Read the model definition and answer for the solid it produces. Units are mm, in the model's axes. A direction names the side the tool comes from. Coordinates: 2 decimals unless noted, no trailing zeros. Write each loop counter-clockwise with the first axis right and the second up, starting at its lowest first coordinate (ties: lowest second). Pieces come first, ordered by that corner, then holes.
Item 1: Straight lines are drawn through the part: probe 1 along Y at (x, z) = (0, 30); probe 2 along X at (y, z) = (-0.75, 15); probe 3 along Z at (x, y) = (-1.5, -0.75). For each, find the intervals that lie inside material, in ascending order.
Item 2: Determine the mould class of faces 4 (the face through (1.926, 0.607, 24.417)), 5 (the face through (0, 0, 12.827)), 6 (the face through (5.474, -3.219, 22.874)), 7 (the face through (0, 0, 0)) for opening direction Y: released by +Y, released by -Y, zero draft, split by the parting line, or undercut.
Item 3: Section C-C (y = -5.25) is taken. Give the vertices of the cut face in (x, z).
Item 4: Section D-D (x = -6) is taken. Give the vertices of the cut face in (y, z).
Item 5: Section A-A (z = 18.5) is taken. Give the vertices of the cut face in (x, y), then the cut area to 3 significant figures.
Item 6: A tool of negligible diameter and unlimited length cuts with its end or side. For faces 1 (the face through (5.525, 3.131, 22.874)), 2 (the face through (0, -6.35, 23)), 3 (the face through (-5.525, -3.131, 22.874)), from which of +Z, -Z, +X, -X, +Y, -Y can it reach the whole face along a straight path? Write none if from no direction.
Item 7: Each of these flat-tipped pins is pushed along its axis until it touches: P1, Ø3, axis at x = 0, y = 0, coming from the +Z side; P2, Ø3, axis at y = 5, z = 6, coming from the +X side; P3, Ø4, axis at x = 4.5, z = 22.5, coming from the +Y side. Where does it stop, or does it pass through?
Item 8: Section B-B (x = 0) is taken. Give the vertices of the cut face in (y, z).
from build123d import *

# Parameters (mm, degrees)
SKETCH2_R           = 7.9248
BOSS_EXTRUDE1_DEPTH = 10.414
BOSS_EXTRUDE2_DEPTH = 25.273
SKETCH4_R           = 2.0193
CUT_EXTRUDE1_DEPTH  = 22.86


with BuildPart() as part:
    # Sketch2 → Boss-Extrude1 (new body)
    with BuildSketch(Plane.XY):
        Circle(SKETCH2_R)
    extrude(amount=BOSS_EXTRUDE1_DEPTH)

    # Sketch3 → Boss-Extrude2 (add)
    with BuildSketch(Plane.XY.offset(10.414)):
        Polygon((7.332348419, 0), (3.666174209, 6.35), (-3.666174209, 6.35), (-7.332348419, 0), (-3.666174209, -6.35), (3.666174209, -6.35), align=None)
    extrude(amount=BOSS_EXTRUDE2_DEPTH)

    # Sketch4 → Cut-Extrude1 (cut)
    with BuildSketch(Plane.XY.offset(35.687)):
        Circle(SKETCH4_R)
    extrude(amount=-CUT_EXTRUDE1_DEPTH, mode=Mode.SUBTRACT)


solid = part.part
Established:
1. probe 1: y = -6.35 to -2.02, 2.02 to 6.35
1. probe 2: x = -6.9 to -1.87, 1.87 to 6.9
1. probe 3: z = 0 to 12.83
2. face 4: undercut
2. face 5: undercut
2. face 6: released by -Y
2. face 7: zero draft
3. outline: (-5.94, 0) - (5.94, 0) - (5.94, 10.41) - (4.3, 10.41) - (4.3, 35.69) - (-4.3, 35.69) - (-4.3, 10.41) - (-5.94, 10.41) - close
4. outline: (-5.18, 0) - (5.18, 0) - (5.18, 10.41) - (2.31, 10.41) - (2.31, 35.69) - (-2.31, 35.69) - (-2.31, 10.41) - (-5.18, 10.41) - close
5. outline: (-7.33, 0) - (-3.67, -6.35) - (3.67, -6.35) - (7.33, 0) - (3.67, 6.35) - (-3.67, 6.35) - close; hole circle Ø4.04 at (0, 0)
5. area: 127 mm2
6. face 1: +Z, +X, +Y
6. face 2: +Z, +X, -X, -Y
6. face 3: +Z, -X, -Y
7. P1: stops at z = 12.83
7. P2: stops at x = 7.11
7. P3: stops at y = 6.35
8. outline: (-7.92, 0) - (7.92, 0) - (7.92, 10.41) - (6.35, 10.41) - (6.35, 35.69) - (2.02, 35.69) - (2.02, 12.83) - (-2.02, 12.83) - (-2.02, 35.69) - (-6.35, 35.69) - (-6.35, 10.41) - (-7.92, 10.41) - close
